from build123d import *

# Parameters (mm, degrees)
BOSS_EXTRUDE1_DEPTH = 6.35
SKETCH9_R           = 2.6
CUT_EXTRUDE1_DEPTH  = 105.776848123


with BuildPart() as part:
    # Sketch1 → Boss-Extrude1 (new body)
    with BuildSketch(Plane(origin=(0, 0, 0), x_dir=(1, 0, 0), z_dir=(0, 1, 0))):
        Polygon((-15.875, 75), (15.875, 75), (72.889405284, -23.751846715), (57.014405284, -51.248153285), (-57.014405284, -51.248153285), (-72.889405284, -23.751846715), align=None)
    extrude(amount=BOSS_EXTRUDE1_DEPTH)

    # Sketch9 → Cut-Extrude1 (cut, through all)
    with BuildSketch(Plane(origin=(0, 6.35, 0), x_dir=(1, 0, 0), z_dir=(0, 1, 0))):
        with Locations(Location((-25.030312278, 49.142819263, 0), (0, 0, 270))):
            Circle(SKETCH9_R)
        with Locations(Location((25.008570083, 49.180192562, 0), (0, 0, 270))):
            Circle(SKETCH9_R)
        with Locations(Location((55.008731986, -2.78123819, 0), (0, 0, 270))):
            Circle(SKETCH9_R)
        with Locations(Location((30.09884337, -46.248153285, 0), (0, 0, 270))):
            Circle(SKETCH9_R)
        with Locations(Location((-55.030188745, -2.818776286, 0), (0, 0, 270))):
            Circle(SKETCH9_R)
        with Locations(Location((-29.90115663, -46.248153285, 0), (0, 0, 270))):
            Circle(SKETCH9_R)
    extrude(amount=-CUT_EXTRUDE1_DEPTH, mode=Mode.SUBTRACT)


solid = part.part
Design review of the part built by this model. Coordinates are the model's own, in mm. Round coordinates to 2 decimals unless told otherwise and drop trailing zeros. Loops run counter-clockwise (first coordinate to the right, second up) from the corner with the lowest first, then second, coordinate; pieces in that order, holes last. Notation, with made-up numbers: (-31, 19.5) - (16, 19.5) arc R14 ccw to (16, 35.5) - close; hole circle Ø8 at (-11.5, 9.5). An arc over 180 degrees is marked (long way). One line per question, with ' | ' between items.
1. We need section D-D, the plane z = -20. State the section outline as (x, y) points.
Results are:
outline: (-47.63, 0) - (47.63, 0) - (47.63, 6.35) - (-47.63, 6.35) - close
2. We need section A-A, the plane z = 3.5. State the section outline as (x, y) points, and give its area (3 significant figures).
Results are:
outline: (-61.2, 0) - (-57.54, 0) - (-57.54, 6.35) - (-61.2, 6.35) - close; (-52.52, 0) - (52.51, 0) - (52.51, 6.35) - (-52.52, 6.35) - close; (57.51, 0) - (61.2, 0) - (61.2, 6.35) - (57.51, 6.35) - close | area: 714 mm²
3. Draft analysis for pull direction X (two halves, no side actions). For faces 1 (the face through (-64.84, 3.13, 37.69)), 2 (the face through (1, 3, 51.248)), 3 (the face through (25.79, 3.22, -46.7)), state which applies: released by +X, released by -X, zero draft, split by the parting line, or undercut.
Results are:
face 1: released by -X | face 2: zero draft | face 3: undercut
4. We need section B-B, the plane y = 4.75. State the section outline as (x, z) points (3 decimals), and give its area (3 significant figures).
Results are:
outline: (-72.889, 23.752) - (-15.875, -75) - (15.875, -75) - (72.889, 23.752) - (57.014, 51.248) - (-57.014, 51.248) - close; hole circle Ø5.2 at (-55.03, 2.819); hole circle Ø5.2 at (-29.901, 46.248); hole circle Ø5.2 at (-25.03, -49.143); hole circle Ø5.2 at (25.009, -49.18); hole circle Ø5.2 at (30.099, 46.248); hole circle Ø5.2 at (55.009, 2.781) | area: 12,200 mm²
5. Clearance check with flat-ended pins moving along their axes: P1, Ø1, axis at y = 2, z = -24.5, coming from the -X side; P2, Ø4, axis at x = -25.03, z = -49.14, coming from the -Y side; P3, Ø2, axis at y = 2, z = -21, coming from the +X side; P4, Ø6, axis at x = 42.5, z = -33.5, coming from the -Y side. State where each tip first meets the part, or that it passes through.
Results are:
P1: stops at x = -45.32 | P2: passes through | P3: stops at x = 47.63 | P4: stops at y = 0
6. For L1, parallel to X at y = 1.5, z = 45.5; L2, parallel to Z at x = -26, y = 5.5; L3, parallel to Z at x = 31, y = 1, list the stretches that pass through material, from the lowest coordinate up. Write a range as [from, to].
Results are:
L1: x = [-60.33, -32.39], [-27.41, 27.61], [32.59, 60.33] | L2: z = [-57.46, -51.56], [-46.73, 51.25] | L3: z = [-48.8, 43.81], [48.69, 51.25]
7. We need section C-C, the plane x = -47.5. State the section outline as (y, z) points, and give its area (3 significant figures).
Results are:
outline: (0, -20.22) - (6.35, -20.22) - (6.35, 51.25) - (0, 51.25) - close | area: 454 mm²
